```python
from build123d import *

# Parameters (mm, degrees)
F1_DEPTH = 2
F0_W     = 5
F0_H     = 1
F0_W_2   = 26.8
F0_H_2   = 50.8
F2_DEPTH = 5
F0_H_3   = 2.5
F3_DEPTH = 15
F4_DEPTH = 25


with BuildPart() as f1:
    # F0 (on Top) → F1 (new body)
    with BuildSketch(Plane.XY):
        Polygon((2.5, 2.5), (13.5, 2.5), (18.5, 2.5), (29.5, 2.5), (29.5, 53.5), (18.5, 53.5), (13.5, 53.5), (2.5, 53.5), align=None)
    extrude(amount=F1_DEPTH)

    # F0 (on Top) → F3 (join)
    with BuildSketch(Plane.XY):
        with Locations((16, 1.25)):
            Rectangle(F0_W, F0_H_3)
        with Locations((16, 54.75)):
            Rectangle(F0_W, F0_H_3)
    extrude(amount=F3_DEPTH)



with BuildPart() as f1b:
    # F0 (on Top) → F1, piece 2 (new body)
    with BuildSketch(Plane.XY):
        with Locations((34.5, 0.5)):
            Rectangle(F0_W, F0_H)
        Polygon((37, 1), (37, 0), (69, 0), (69, 56), (37, 56), align=None)
        with Locations((53, 28)):
            Rectangle(F0_W_2, F0_H_2, mode=Mode.SUBTRACT)
    extrude(amount=F1_DEPTH)

    # F0 (on Top) → F2 (join)
    with BuildSketch(Plane.XY):
        with Locations((53, 28)):
            Rectangle(F0_W_2, F0_H_2)
    extrude(amount=F2_DEPTH)


with BuildPart() as f1_1:
    add(f1.part)

    add(f1b.part)  # F4 merges F1b
    # F0 (on Top) → F4 (join)
    with BuildSketch(Plane.XY):
        Polygon((0, 56), (0, 0), (13.5, 0), (13.5, 2.5), (2.5, 2.5), (2.5, 53.5), (13.5, 53.5), (13.5, 56), align=None)
        Polygon((18.5, 2.5), (18.5, 0), (32, 0), (32, 1), (32, 56), (18.5, 56), (18.5, 53.5), (29.5, 53.5), (29.5, 2.5), align=None)
    extrude(amount=F4_DEPTH)


solid = f1_1.part
```
Geometry check sheet. Reference: the model listing, model coordinates, mm. A direction names the side the tool comes from. Coordinates: 2 decimals unless noted, no trailing zeros. Write each loop counter-clockwise with the first axis right and the second up, starting at its lowest first coordinate (ties: lowest second). Pieces come first, ordered by that corner, then holes. Notation, with made-up numbers: M -21,38.25 L 25,38.25 A9 ccw 25,46.25 Z; hole C 6,18.5 d4. An arc over 180 degrees is marked long. Answer as a JSON object with one key per item and string values.
1. Draft check along Y on faces 5 (the flat face through (16, 56, 12)), 6 (the flat face through (16, 53.5, 13)), 7 (the flat face through (18.5, 55, 20)). Enter one of: released by +Y, released by -Y, zero draft, split by the parting line, or undercut.
Answers below:
{"face 5": "released by +Y", "face 6": "undercut", "face 7": "zero draft"}
2. Tool access check on faces 1 (the flat face through (29.5, 28, 13)), 2 (the flat face through (53, 2.6, 3)), 3 (the flat face through (37, 29, 1)), 4 (the flat face through (39.6, 28, 3)). Record the directions out of +Z, -Z, +X, -X, +Y, -Y that give a thin tool (end or side, any length) a straight path to the whole face; none if there is none.
Answers below:
{"face 1": "+Z", "face 2": "+Z, +X, -Y", "face 3": "+Z, -Z, +Y", "face 4": "+Z, +Y, -Y"}
3. Section check B-B, the plane y = 25. Enter the section's corners in (x, z), plus the area to 3 significant figures.
Answers below:
{"outline": "M 0,0 L 32,0 L 32,25 L 29.5,25 L 29.5,2 L 2.5,2 L 2.5,25 L 0,25 Z; M 37,0 L 69,0 L 69,2 L 66.4,2 L 66.4,5 L 39.6,5 L 39.6,2 L 37,2 Z", "area": "323 mm²"}
4. Scan lines: L1, parallel to Y at x = 23, z = 12; L2, parallel to X at y = 32, z = 10; L3, parallel to Z at x = 66.5, y = 52. Record each from-to range of solid material in increasing order.
Answers below:
{"L1": "y = 0 to 2.5, 53.5 to 56", "L2": "x = 0 to 2.5, 29.5 to 32", "L3": "z = 0 to 2"}
5. Section check D-D, the plane z = 18.5. Enter the section's corners in (x, y).
Answers below:
{"outline": "M 0,0 L 13.5,0 L 13.5,2.5 L 2.5,2.5 L 2.5,53.5 L 13.5,53.5 L 13.5,56 L 0,56 Z; M 18.5,0 L 32,0 L 32,56 L 18.5,56 L 18.5,53.5 L 29.5,53.5 L 29.5,2.5 L 18.5,2.5 Z"}
6. Section check C-C, the plane z = 11.5. Enter the section's corners in (x, y), plus the area to 3 significant figures.
Answers below:
{"outline": "M 0,0 L 32,0 L 32,56 L 0,56 Z; hole M 2.5,2.5 L 29.5,2.5 L 29.5,53.5 L 2.5,53.5 Z", "area": "415 mm²"}
7. Go/stop test with flat-tipped pins: pin 1 Ø5 at (x, y) = (61.5, 37.5) entering from -Z; pin 2 Ø1.5 at (y, z) = (17.5, 3.5) entering from +X; pin 3 Ø3 at (y, z) = (54.5, 19.5) entering from +X; pin 4 Ø8 at (x, y) = (49, 22.5) entering from +Z. Record where each tip stops, or that it passes through.
Answers below:
{"pin 1": "stops at z = 0", "pin 2": "stops at x = 66.4", "pin 3": "stops at x = 32", "pin 4": "stops at z = 5"}
8. Section check A-A, the plane z = 2.75. Enter the section's corners in (x, y).
Answers below:
{"outline": "M 0,0 L 32,0 L 32,56 L 0,56 Z; M 39.6,2.6 L 66.4,2.6 L 66.4,53.4 L 39.6,53.4 Z; hole M 2.5,2.5 L 29.5,2.5 L 29.5,53.5 L 2.5,53.5 Z"}
